Geometry check sheet. Reference: the model listing, model coordinates, mm. A direction names the side the tool comes from. Coordinates: 2 decimals unless noted, no trailing zeros. Order: outer loops, then holes, each group sorted by start corner. A loop starts at its lowest first (then second) coordinate and runs counter-clockwise, first axis right, second up. Notation, with made-up numbers: (-27.75, 1.5) - (-13.75, 1.5) arc R23 cw to (-13.75, 33.5) - close; hole circle Ø5 at (3.5, -32). An arc over 180 degrees is marked (long way). Use CSV: the item, a comma, the result in double quotes. Start each with the question number.
1) Tool access check on faces 1 (the flat face through (103, 127, 114)), 2 (the cylindrical face through (304.775, 2.234, 12.522)), 3 (the flat face through (100, -127, 114)), 4 (the cylindrical face through (273.033, 1.536, 113.767)). Record the directions out of +Z, -Z, +X, -X, +Y, -Y that give a thin tool (end or side, any length) a straight path to the whole face; none if there is none.
2) Sectioned sample at B-B, the plane z = 15. Record the cut outline in (x, y), and give its area (3 significant figures).
3) Thickness scan on probe 1 along Y at (x, z) = (203, 89); probe 2 along X at (y, z) = (2, 77); probe 3 along Y at (x, z) = (122.5, 102). Record the ranges inside material, lowest first. Write a range as [from, to].
4) Sectioned sample at D-D, the plane y = -42.5. Record the cut outline in (x, z), and give its area (3 significant figures).
5) Draft check along Y on faces 5 (the cylindrical face through (-2.75, -12.4, 81.75)), 6 (the flat face through (10.6, 23.3, 152.4)), 7 (the cylindrical face through (406.35, -4.47, 37.57)), 8 (the flat face through (99, -1, 25.4)). Enter one of: released by +Y, released by -Y, zero draft, split by the parting line, or undercut.
6) Sectioned sample at A-A, the plane z = 114.5. Record the cut outline in (x, y).
7) Sectioned sample at C-C, the plane x = 91. Record the cut outline in (y, z).
8) Depth check by flat-ended pin: P1, Ø10, axis at x = 230.5, z = 58.5, coming from the -Y side; P2, Ø8, axis at y = -51.5, z = 60, coming from the -X side; P3, Ø23, axis at x = 0, y = 0, coming from the -Z side; P4, Ø23, axis at x = 84, z = 120, coming from the -Y side. Enter the tip coordinate at first touch or a pass-through.
from build123d import *

# Parameters (mm, degrees)
F1_DEPTH = 76.2
F2_R     = 50.8
F2_R_2   = 25.4
F2_R_3   = 12.7
F3_DEPTH = 76.2
F4_SIZE  = 12.7
F6_DEPTH = 25.4
F7_DEPTH = 50.8


with BuildPart() as f1:
    # F0 (on Top) → F1 (new body)
    with BuildSketch(Plane.XY):
        with BuildLine():
            Line((203.2, 203.2), (0, 203.2))
            ThreePointArc((0, 203.2), (-203.2, 0), (0, -203.2))
            Line((0, -203.2), (203.2, -203.2))
            ThreePointArc((203.2, -203.2), (406.4, 0), (203.2, 203.2))
        make_face()
    extrude(amount=F1_DEPTH)

    # F2 (on face) → F3 (join)
    with BuildSketch(Plane.XY.offset(76.2)):
        with BuildLine():
            Line((0, -127), (203.2, -127))
            ThreePointArc((203.2, -127), (330.2, 0), (203.2, 127))
            Line((203.2, 127), (0, 127))
            ThreePointArc((0, 127), (-127, 0), (0, -127))
        make_face()
        with BuildLine():
            ThreePointArc((0, -69.85), (-69.85, 0), (0, 69.85))
            Line((0, 69.85), (203.2, 69.85))
            ThreePointArc((203.2, 69.85), (273.05, 0), (203.2, -69.85))
            Line((203.2, -69.85), (0, -69.85))
        make_face(mode=Mode.SUBTRACT)
        Circle(F2_R)
        Circle(F2_R_2, mode=Mode.SUBTRACT)
        with Locations((203.2, 0)):
            Circle(F2_R)
        with Locations((203.2, 0)):
            Circle(F2_R_2, mode=Mode.SUBTRACT)
        Circle(F2_R_2)
        Circle(F2_R_3, mode=Mode.SUBTRACT)
        with Locations((203.2, 0)):
            Circle(F2_R_2)
        with Locations((203.2, 0)):
            Circle(F2_R_3, mode=Mode.SUBTRACT)
    extrude(amount=F3_DEPTH)

    # F4
    f4_edges = [f1.edges().sort_by_distance(p)[0] for p in [
        (-12.7, 0, 152.4),
        (190.5, 0, 152.4),
    ]]
    chamfer(f4_edges, length=F4_SIZE)

    # F5 (on face) → F6 (cut)
    with BuildSketch(Plane(origin=(0, 0, 0), x_dir=(1, 0, 0), z_dir=(0, 0, -1))):
        with BuildLine():
            Line((203.2, 101.6), (0, 101.6))
            ThreePointArc((0, 101.6), (-101.6, 0), (0, -101.6))
            Line((0, -101.6), (203.2, -101.6))
            ThreePointArc((203.2, -101.6), (304.8, 0), (203.2, 101.6))
        make_face()
    extrude(amount=-F6_DEPTH, mode=Mode.SUBTRACT)

    # F7 (cut): faces of the model
    f7_faces = [f1.faces().sort_by_distance(p)[0] for p in [
        (0, 0, 76.2),
        (203.2, 0, 76.2),
    ]]
    extrude(f7_faces, amount=-F7_DEPTH, mode=Mode.SUBTRACT)


solid = f1.part
Evaluation:
1,face 1,"+Z, +X, -X, +Y"
1,face 2,"-Z"
1,face 3,"+Z, +X, -X, -Y"
1,face 4,"+Z"
2,outline,"(0, -203.2) - (203.2, -203.2) arc R203.2 ccw to (203.2, 203.2) - (0, 203.2) arc R203.2 ccw to start; hole (0, -101.6) - (203.2, -101.6) arc R101.6 ccw to (203.2, 101.6) - (0, 101.6) arc R101.6 ccw to start"
2,area,"139,000 mm²"
3,probe 1,"[-127, -69.85], [-50.8, -12.7], [12.7, 50.8], [69.85, 127]"
3,probe 2,"[-126.98, -69.82], [-50.76, -12.54], [12.54, 50.76], [152.44, 190.66], [215.74, 253.96], [273.02, 330.18]"
3,probe 3,"[-127, -69.85], [69.85, 127]"
4,outline,"(-198.71, 0) - (-92.28, 0) - (-92.28, 25.4) - (295.48, 25.4) - (295.48, 0) - (401.91, 0) - (401.91, 76.2) - (322.88, 76.2) - (322.88, 152.4) - (258.63, 152.4) - (258.63, 76.2) - (231.03, 76.2) - (231.03, 152.4) - (175.37, 152.4) - (175.37, 76.2) - (27.83, 76.2) - (27.83, 152.4) - (-27.83, 152.4) - (-27.83, 76.2) - (-55.43, 76.2) - (-55.43, 152.4) - (-119.68, 152.4) - (-119.68, 76.2) - (-198.71, 76.2) - close"
4,area,"54,200 mm²"
5,face 5,"undercut"
5,face 6,"zero draft"
5,face 7,"split by the parting line"
5,face 8,"undercut"
6,outline,"circle Ø101.6 at (0, 0); (0, -127) - (203.2, -127) arc R127 ccw to (203.2, 127) - (0, 127) arc R127 ccw to start; circle Ø101.6 at (203.2, 0); hole circle Ø25.4 at (0, 0); hole (0, -69.85) - (203.2, -69.85) arc R69.85 ccw to (203.2, 69.85) - (0, 69.85) arc R69.85 ccw to start; hole circle Ø25.4 at (203.2, 0)"
7,outline,"(-203.2, 0) - (-101.6, 0) - (-101.6, 25.4) - (101.6, 25.4) - (101.6, 0) - (203.2, 0) - (203.2, 76.2) - (127, 76.2) - (127, 152.4) - (69.85, 152.4) - (69.85, 76.2) - (-69.85, 76.2) - (-69.85, 152.4) - (-127, 152.4) - (-127, 76.2) - (-203.2, 76.2) - close"
8,P1,"y = -201.97"
8,P2,"x = -197.57"
8,P3,"through"
8,P4,"y = -127"
